Part model, mm, in its own coordinate system. Round coordinates to 2 decimals unless told otherwise and drop trailing zeros. Write each loop counter-clockwise with the first axis right and the second up, starting at its lowest first coordinate (ties: lowest second). Pieces come first, ordered by that corner, then holes. Notation, with made-up numbers: (-3.5, 22.25) -> (29.5, 22.25) arc R23 cw to (29.5, 47.25) -> close; hole circle Ø9 at (11.5, -8.5). An arc over 180 degrees is marked (long way). Return JSON: item names as keys, results as strings. Group by question number.
(1) Saw through at C-C (x = -7). List the corners of the cut face in (y, z) (3 decimals).
(2) Drop flat-ended pins along their axis: pin 1 Ø1 at (y, z) = (159.5, -6) entering from +X; pin 2 Ø2 at (x, z) = (-41.5, 3.5) entering from -Y; pin 3 Ø0.6 at (y, z) = (160, -7.5) entering from -X. Give the stop position or say it passes through.
(3) Saw through at A-A (z = 9). List the corners of the cut face in (x, y) (3 decimals), plus the area to 3 significant figures.
(4) Drill centre line: L1, parallel to Y at x = 56, z = 1.5. Where is it in solid material? Low to high. Write a range as from..to.
(5) Saw through at B-B (x = 25.5). List the corners of the cut face in (y, z) (3 decimals).
(6) Mould opens along X. For faces 1 (the flat face through (-17, 160.65, -7)), 2 (the flat face through (-1, 0, 0)), 3 (the flat face through (-61.425, 78, 0)) say: +X half, -X half, draft (parallel to the pull), parting line (faces both ways), or undercut.
from build123d import *

# Parameters (mm, degrees)
F0_W     = 122.85
F0_H     = 34.45
F2_DEPTH = 158.65
F3_DEPTH = 2
F7_DEPTH = 2


with BuildPart() as f2:
    # F0 (on Front) → F2 (new body)
    with BuildSketch(Plane.XZ):
        Rectangle(F0_W, F0_H)
    extrude(amount=-F2_DEPTH)

    # F1 (on Front) → F3 (join)
    with BuildSketch(Plane.XZ):
        Polygon((-46.840929, -11.1012), (-42.385265, -8.427801), (-42.472665, -3.232384), (-47.015728, -0.710365), (-51.471391, -3.383764), (-51.383992, -8.579181), align=None)
        Polygon((-23.726419, -11.12884), (-19.144532, -8.678063), (-18.976023, -3.484643), (-23.389402, -0.742001), (-27.97129, -3.192778), (-28.139798, -8.386198), align=None)
        Polygon((23.452608, -10.195813), (27.906654, -7.519719), (27.816112, -2.324356), (23.271524, 0.194914), (18.817478, -2.48118), (18.90802, -7.676543), align=None)
    extrude(amount=F3_DEPTH)

    # F6 (on face) → F7 (join)
    with BuildSketch(Plane(origin=(0, 158.65, 0), x_dir=(-1, 0, 0), z_dir=(0, 1, 0))):
        Polygon((37.586212, -9.593843), (42.029951, -12.287017), (46.584177, -9.785213), (46.694665, -4.590235), (42.250926, -1.897062), (37.696699, -4.398866), align=None)
        Polygon((16.800624, -12.363649), (21.244363, -9.670475), (21.244363, -4.474323), (16.690137, -1.972519), (12.246398, -4.665692), (12.246398, -9.861845), align=None)
        Polygon((-21.518063, -9.199932), (-17.018063, -11.798008), (-12.518063, -9.199932), (-12.518063, -4.00378), (-17.018063, -1.405703), (-21.518063, -4.00378), align=None)
        Polygon((-42.418962, -1.405703), (-46.918962, -4.00378), (-46.918962, -9.199932), (-42.418962, -11.798008), (-37.918962, -9.199932), (-37.918962, -4.00378), align=None)
    extrude(amount=F7_DEPTH)


solid = f2.part
Computed values:
{
 "1": {"outline": "(0, -17.225) -> (158.65, -17.225) -> (158.65, 17.225) -> (0, 17.225) -> close"},
 "2": {"pin 1": "x = 46.92", "pin 2": "y = 0", "pin 3": "x = -46.64"},
 "3": {"outline": "(-61.425, 0) -> (61.425, 0) -> (61.425, 158.65) -> (-61.425, 158.65) -> close", "area": "19,500 mm2"},
 "4": {"L1": "0..158.65"},
 "5": {"outline": "(-2, -8.966) -> (0, -8.966) -> (0, -17.225) -> (158.65, -17.225) -> (158.65, 17.225) -> (0, 17.225) -> (0, -1.04) -> (-2, -1.04) -> close"},
 "6": {"face 1": "draft", "face 2": "undercut", "face 3": "-X half"}
}
